```python
from build123d import *

# Parameters (mm, degrees)
SKETCH_1_R      = 1.5
EXTRUDE_1_DEPTH = 2


with BuildPart() as part:
    # 草图1 → 凸台-拉伸1 (new body)
    with BuildSketch(Plane(origin=(0, 0, 0), x_dir=(0, 0, -1), z_dir=(1, 0, 0))):
        with BuildLine():
            ThreePointArc((-2.999407201, 0.059635923), (0, -3), (2.999407201, 0.059635923))
            ThreePointArc((2.999407201, 0.059635923), (3.053738623, 42.383739267), (4.898951428, 84.667635321))
            ThreePointArc((4.898951428, 84.667635321), (4.573390935, 85.168972903), (4, 85))
            ThreePointArc((4, 85), (0, 83), (-4, 85))
            ThreePointArc((-4, 85), (-4.573390935, 85.168972903), (-4.898951428, 84.667635321))
            ThreePointArc((-4.898951428, 84.667635321), (-3.053738623, 42.383739267), (-2.999407201, 0.059635923))
        make_face()
        Circle(SKETCH_1_R, mode=Mode.SUBTRACT)
        with Locations((0, 80)):
            Circle(SKETCH_1_R, mode=Mode.SUBTRACT)
        with Locations((0, 60)):
            Circle(SKETCH_1_R, mode=Mode.SUBTRACT)
    extrude(amount=EXTRUDE_1_DEPTH)


solid = part.part
```
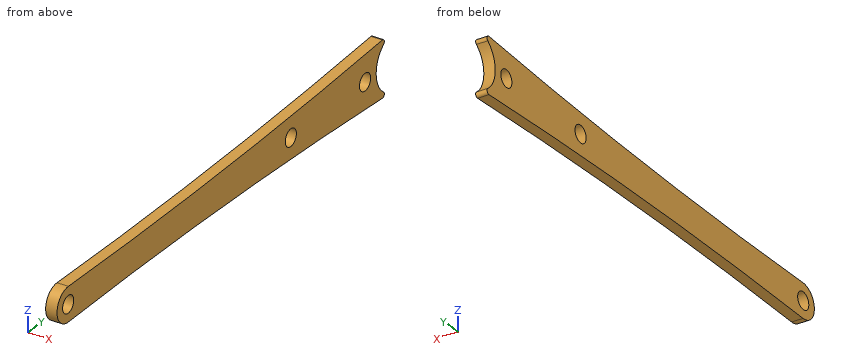
Part model, mm, in its own coordinate system. Coordinates: 2 decimals unless noted, no trailing zeros. Order: outer loops, then holes, each group sorted by start corner. A loop starts at its lowest first (then second) coordinate and runs counter-clockwise, first axis right, second up. Notation, with made-up numbers: (64.5, 38) - (106.5, 38) arc R19 ccw to (106.5, 57) - close; hole circle Ø3 at (82, -30). An arc over 180 degrees is marked (long way). Return JSON: item names as keys, results as strings. Group by question number.
Item 1: Pin check, flat tip, straight feed: pin 1 (2.5 mm diameter, centred on y = 60, z = 0, fed in from +X). Stop position of the tip, or through.
Item 2: Cut at D-D (y = 80). List the corners of the cut face in (x, z).
Item 3: Cut at A-A (z = 0). List the corners of the cut face in (x, y).
Item 4: Drill centre lines: probe 1 along Y at (x, z) = (0.55, 0); probe 2 along Y at (x, z) = (1.85, -1); probe 3 along Z at (x, y) = (1.4, 80). Where is each one in solid material? Low to high. Write a range as from..to.
Item 5: Cut at C-C (x = 0.4). List the corners of the cut face in (y, z).
Check values:
{
 "1": {"pin 1": "passes through"},
 "2": {"outline": "(0, -4.61) - (2, -4.61) - (2, -1.5) - (0, -1.5) - close; (0, 1.5) - (2, 1.5) - (2, 4.61) - (0, 4.61) - close"},
 "3": {"outline": "(0, -3) - (2, -3) - (2, -1.5) - (0, -1.5) - close; (0, 1.5) - (2, 1.5) - (2, 58.5) - (0, 58.5) - close; (0, 61.5) - (2, 61.5) - (2, 78.5) - (0, 78.5) - close; (0, 81.5) - (2, 81.5) - (2, 83) - (0, 83) - close"},
 "4": {"probe 1": "y = -3..-1.5, 1.5..58.5, 61.5..78.5, 81.5..83", "probe 2": "y = -2.83..-1.12, 1.12..58.88, 61.12..78.88, 81.12..83.1", "probe 3": "z = -4.61..-1.5, 1.5..4.61"},
 "5": {"outline": "(0.06, -3) arc R1000 cw to (84.67, -4.9) arc R0.5 ccw to (85, -4) arc R5 cw to (85, 4) arc R0.5 ccw to (84.67, 4.9) arc R1000 cw to (0.06, 3) arc R3 ccw (long way) to start; hole circle Ø3 at (0, 0); hole circle Ø3 at (60, 0); hole circle Ø3 at (80, 0)"}
}
